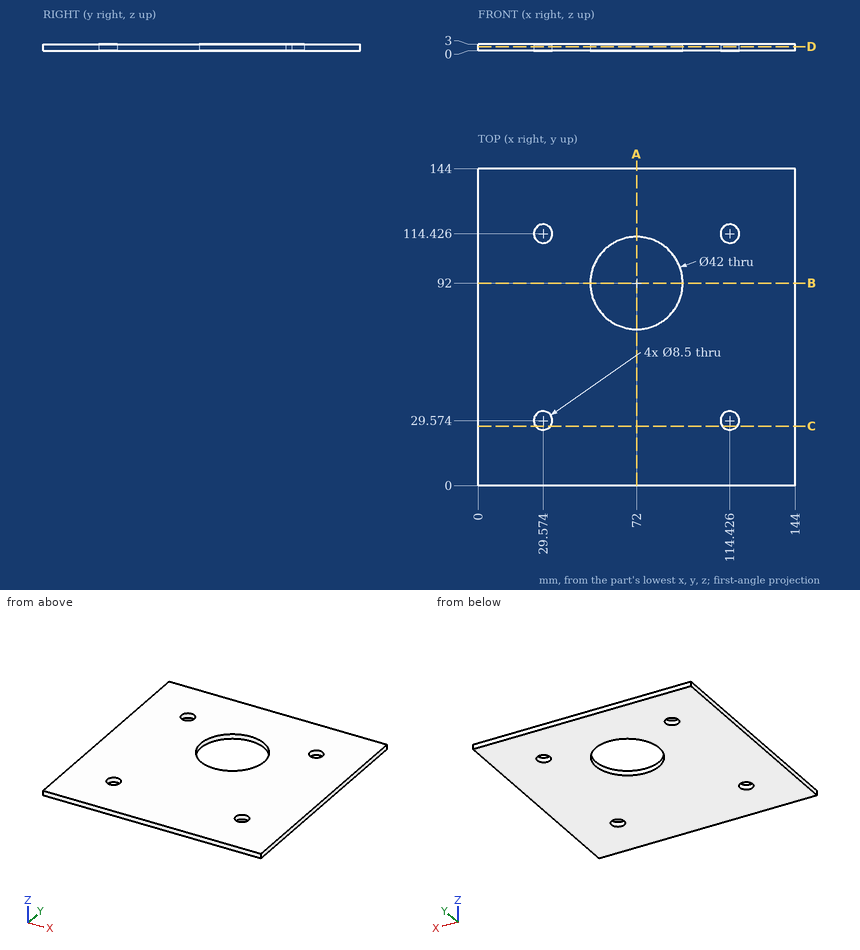
Here's the drawing with two shaded views (mm, measured from the low corner). I have some questions. Coordinates: 2 decimals unless noted, no trailing zeros. Loops run counter-clockwise (first coordinate to the right, second up) from the corner with the lowest first, then second, coordinate; pieces in that order, holes last. Notation, with made-up numbers: (14.25, 83.25) - (53.25, 83.25) arc R19 ccw to (53.25, 90.25) - close; hole circle Ø8 at (-39.75, 84.25). An arc over 180 degrees is marked (long way). Answer as CSV lines item,"result". Start each with the question number.
1) I need wall thicknesses on line 1 (X direction, y = 91.5, z = 2.95); line 2 (Y direction, x = 111.5, z = 1.55) (1 decimal); line 3 (Y direction, x = 30.5, z = 1.4) (1 decimal). Which ranges of each line are inside material? Lowest first, please. Write a range as from..to.
2) Suppose I cut it at C-C (y = 27). Please give me the cut outline in (x, z) (1 decimal).
3) Suppose I cut it at A-A (x = 72). Please give me the cut outline in (y, z), plus the area to 3 significant figures.
4) Suppose I cut it at B-B (y = 92). Please give me the cut outline in (x, z), plus the area to 3 significant figures.
5) Suppose I cut it at D-D (z = 1.85). Please give me the cut outline in (x, y).
Check result:
1,line 1,"x = 0..51.01, 92.99..144"
1,line 2,"y = 0..26.5, 32.7..111.3, 117.5..144"
1,line 3,"y = 0..25.4, 33.7..110.3, 118.6..144"
2,outline,"(0, 0) - (26.2, 0) - (26.2, 3) - (0, 3) - close; (33, 0) - (111, 0) - (111, 3) - (33, 3) - close; (117.8, 0) - (144, 0) - (144, 3) - (117.8, 3) - close"
3,outline,"(0, 0) - (71, 0) - (71, 3) - (0, 3) - close; (113, 0) - (144, 0) - (144, 3) - (113, 3) - close"
3,area,"306 mm²"
4,outline,"(0, 0) - (51, 0) - (51, 3) - (0, 3) - close; (93, 0) - (144, 0) - (144, 3) - (93, 3) - close"
4,area,"306 mm²"
5,outline,"(0, 0) - (144, 0) - (144, 144) - (0, 144) - close; hole circle Ø8.5 at (29.57, 29.57); hole circle Ø8.5 at (29.57, 114.43); hole circle Ø42 at (72, 92); hole circle Ø8.5 at (114.43, 29.57); hole circle Ø8.5 at (114.43, 114.43)"
